from build123d import *

# Parameters (mm, degrees)
SKETCH1_R           = 7.5
BOSS_EXTRUDE1_DEPTH = 2
SKETCH2_W           = 5
SKETCH2_H           = 6.920756948
BOSS_EXTRUDE2_DEPTH = 1.5
SKETCH3_W           = 7
SKETCH3_H           = 2
BOSS_EXTRUDE3_DEPTH = 3


with BuildPart() as part:
    # Sketch1 → Boss-Extrude1 (new body)
    with BuildSketch(Plane.XY):
        Circle(SKETCH1_R)
    extrude(amount=BOSS_EXTRUDE1_DEPTH)

    # Sketch2 → Boss-Extrude2 (add)
    with BuildSketch(Plane.XY.offset(2)):
        with Locations((0.310238116, 0.506092566)):
            Rectangle(SKETCH2_W, SKETCH2_H)
    extrude(amount=BOSS_EXTRUDE2_DEPTH)

    # Sketch3 → Boss-Extrude3 (add)
    with BuildSketch(Plane(origin=(0, 0, 0), x_dir=(-1, 0, 0), z_dir=(0, 0, -1))):
        with Locations((0, 4.5)):
            Rectangle(SKETCH3_W, SKETCH3_H)
    extrude(amount=BOSS_EXTRUDE3_DEPTH)


solid = part.part
Design review of the part built by this model. Coordinates are the model's own, in mm. A direction names the side the tool comes from. Round coordinates to 2 decimals unless told otherwise and drop trailing zeros. Write each loop counter-clockwise with the first axis right and the second up, starting at its lowest first coordinate (ties: lowest second). Pieces come first, ordered by that corner, then holes. Notation, with made-up numbers: (6, -33.75) - (10, -33.75) arc R28 ccw to (10, -11.75) - close; hole circle Ø8 at (-24.5, 42.5). An arc over 180 degrees is marked (long way). Use a Markdown table: item, result. Add a question column.
1. Clearance check with flat-ended pins moving along their axes: pin 1 (1.6 mm diameter, centred on y = 4.5, z = -1, fed in from -X); pin 2 (5 mm diameter, centred on x = 5, y = -2.5, fed in from -Z); pin 3 (3.5 mm diameter, centred on x = 1, z = -2, fed in from +Y). State where each tip first meets the part, or that it passes through.
2. We need section D-D (z = 1.25). State the section outline as (x, y) points, then the cut area to 3 significant figures.
3. We need section C-C (z = -2.5). State the section outline as (x, y) points.
4. Wall thickness on probe 1 along Z at (x, y) = (3.75, -1.5); probe 2 along X at (y, z) = (5, -2); probe 3 along Z at (x, y) = (0.5, 2.25): over which ranges is each line inside the solid? List them lowest first.
5. We need section A-A (y = 0). State the section outline as (x, z) points, then the cut area to 3 significant figures.
6. For faces 1 (the face through (3.5, 4, -1)), 2 (the face through (2.81, 0, 3)), 3 (the face through (0, -2.954, 3)), list the 3-axis set-ups (+Z, -Z, +X, -X, +Y, -Y) from which the entire face can be reached by the end or side of a thin tool; tool diameter is ignored.
7. We need section B-B (x = 0). State the section outline as (y, z) points.
Output:
| question | item | result |
|---|---|---|
| 1 | pin 1 | stops at x = -3.5 |
| 1 | pin 2 | stops at z = 0 |
| 1 | pin 3 | stops at y = 5.5 |
| 2 | outline | circle Ø15 at (0, 0) |
| 2 | area | 177 mm2 |
| 3 | outline | (-3.5, 3.5) - (3.5, 3.5) - (3.5, 5.5) - (-3.5, 5.5) - close |
| 4 | probe 1 | z = 0 to 2 |
| 4 | probe 2 | x = -3.5 to 3.5 |
| 4 | probe 3 | z = 0 to 3.5 |
| 5 | outline | (-7.5, 0) - (7.5, 0) - (7.5, 2) - (2.81, 2) - (2.81, 3.5) - (-2.19, 3.5) - (-2.19, 2) - (-7.5, 2) - close |
| 5 | area | 37.5 mm2 |
| 6 | face 1 | -Z, +X, +Y, -Y |
| 6 | face 2 | +Z, +X, +Y, -Y |
| 6 | face 3 | +Z, +X, -X, -Y |
| 7 | outline | (-7.5, 0) - (3.5, 0) - (3.5, -3) - (5.5, -3) - (5.5, 0) - (7.5, 0) - (7.5, 2) - (3.97, 2) - (3.97, 3.5) - (-2.95, 3.5) - (-2.95, 2) - (-7.5, 2) - close |
